from build123d import *

# Parameters (mm, degrees)
F1_DEPTH = 40
F0_R     = 10
F2_DEPTH = 15
F4_R     = 19.99999
F5_R     = 10
F6_DEPTH = 15


# Not quite as in the source:
# - a fillet or chamfer is up to 0.001 mm smaller than in the source, because OpenCascade refuses the exact size


with BuildPart() as f1:
    # F0 (on Front) → F1 (new body)
    with BuildSketch(Plane.XZ):
        Polygon((0, 20), (0, 0), (80, 0), (80, 60), (65, 60), (65, 20), (40, 20), align=None)
    extrude(amount=F1_DEPTH)

    # F0 (on Front) → F2 (join)
    with BuildSketch(Plane.XZ):
        with BuildLine():
            Line((0, 40), (0, 20))
            Line((0, 20), (40, 20))
            Line((40, 20), (40, 40))
            ThreePointArc((40, 40), (20, 60), (0, 40))
        make_face()
        with Locations((20, 40)):
            Circle(F0_R, mode=Mode.SUBTRACT)
    extrude(amount=F2_DEPTH)

    # F4 (radius 20 in the source; OpenCascade refuses exactly that, so slightly less here)
    f4_edges = [f1.edges().sort_by_distance(p)[0] for p in [
        (72.5, -40, 60),
        (72.5, 0, 60),
    ]]
    fillet(f4_edges, radius=F4_R)

    # F5 (on face) → F6 (cut, through all)
    with BuildSketch(Plane.YZ.offset(80)):
        with Locations((-20, 40)):
            Circle(F5_R)
    extrude(amount=-F6_DEPTH, mode=Mode.SUBTRACT)


solid = f1.part
Model file for the job. Use its own axes, mm. A direction names the side the tool comes from. Give positions to 0.01 mm unless a question says otherwise; leave off trailing zeros. Loops run counter-clockwise (first coordinate to the right, second up) from the corner with the lowest first, then second, coordinate; pieces in that order, holes last. Notation, with made-up numbers: (-23, 54.5) - (25, 54.5) arc R24 cw to (25, 67.5) - close; hole circle Ø10 at (70, -5.5). An arc over 180 degrees is marked (long way). Use one line per item in the form item = value.
(1) Cut at C-C (y = -13). Give the cut face in (x, z) (3 decimals).
Determined:
outline = (0, 0) - (80, 0) - (80, 32.859) - (65, 32.859) - (65, 20) - (40, 20) - (40, 40) arc R20 ccw to (0, 40) - close; (65, 47.141) - (80, 47.141) - (80, 58.735) - (65, 58.735) - close; hole circle Ø20 at (20, 40)
(2) Drill centre lines: L1, parallel to Z at x = 73.5, y = -20; L2, parallel to Z at x = 22.5, y = -21; L3, parallel to Y at x = 38.5, z = 31. Where is each one in solid material? Low to high.
Determined:
L1 = 0 to 30, 50 to 60
L2 = 0 to 20
L3 = -15 to 0
(3) Pull direction Z, two halves, no side cores. Call faces 1 (the face through (72.395, -5.703, 53.986)), 2 (the face through (72.605, -15.386, 31.128)), 3 (the face through (20, -15, 27)): pulls with the +Z half, pulls with the -Z half, needs draft (parallel to the pull), parting line crosses it, or undercut.
Determined:
face_1 = pulls with the +Z half
face_2 = undercut
face_3 = needs draft
(4) Drop flat-ended pins along their axis: P1, Ø4, axis at x = 17, y = -16.5, coming from the +Z side; P2, Ø4, axis at x = 19, y = -30.5, coming from the +Z side; P3, Ø20, axis at y = -26, z = 36.5, coming from the -X side; P4, Ø16, axis at x = 20, z = 40, coming from the -Y side (3 decimals). Give the stop position or say it passes through.
Determined:
P1 = 59.93
P2 = 20
P3 = 65
P4 = through
(5) Cut at A-A (x = 20). Give the cut face in (y, z), then the cut area to 3 significant figures.
Determined:
outline = (-40, 0) - (0, 0) - (0, 30) - (-15, 30) - (-15, 20) - (-40, 20) - close; (-15, 50) - (0, 50) - (0, 60) - (-15, 60) - close
area = 1,100 mm^2
(6) Cut at D-D (z = 52.5). Give the cut face in (x, y).
Determined:
outline = (4.39, -15) - (35.61, -15) - (35.61, 0) - (4.39, 0) - close; (65, -35.61) - (80, -35.61) - (80, -4.39) - (65, -4.39) - close
(7) 3-axis set-ups, long thin cutter, end or side, ignore diameter. For faces 4 (the face through (40, -7, 30)), 5 (the face through (39, -20, 0)): which of +Z, -Z, +X, -X, +Y, -Y reach the whole face in a straight line?
Determined:
face_4 = +Z, +Y, -Y
face_5 = -Z, +X, -X, +Y, -Y
